```python
from build123d import *

# Parameters (mm, degrees)
SKETCH1_W               = 15
SKETCH1_H               = 22
SKETCH1_R               = 1.3
SKETCH1_R_2             = 0.5
BOSS_EXTRUDE1_DEPTH     = 1.55
SKETCH2_W               = 4.3
SKETCH2_H               = 5.2
BOSS_EXTRUDE2_DEPTH     = 1
SKETCH4_W               = 22
SKETCH4_H               = 1.55
BOSS_EXTRUDE3_DEPTH     = 13
SKETCH6_W               = 5
SKETCH6_H               = 20
BOSS_EXTRUDE4_DEPTH     = 2.4
BOSS_EXTRUDE5_START     = -5
SKETCH7_R               = 0.45
BOSS_EXTRUDE5_DEPTH     = 11
LPATTERN1_COUNT         = 4
LPATTERN1_PITCH         = 2.54
LPATTERN1_COUNT_DIR2    = 2
LPATTERN1_PITCH_DIR2    = 2.54
MIRROR1_START           = -5
MIRROR1_COPY_1_SKETCH_R = 0.45
MIRROR1_COPY_1_DEPTH    = 11
MIRROR1_COPY_2_SKETCH_R = 0.45
MIRROR1_COPY_2_DEPTH    = 11
MIRROR1_COPY_3_SKETCH_R = 0.45
MIRROR1_COPY_3_DEPTH    = 11
MIRROR1_COPY_4_SKETCH_R = 0.45
MIRROR1_COPY_4_DEPTH    = 11
MIRROR1_COPY_5_SKETCH_R = 0.45
MIRROR1_COPY_5_DEPTH    = 11
MIRROR1_COPY_6_SKETCH_R = 0.45
MIRROR1_COPY_6_DEPTH    = 11
MIRROR1_COPY_7_SKETCH_R = 0.45
MIRROR1_COPY_7_DEPTH    = 11


with BuildPart() as part:
    # Sketch1 → Boss-Extrude1 (new body)
    with BuildSketch(Plane(origin=(0, 0, 0), x_dir=(1, 0, 0), z_dir=(0, 1, 0))):
        Rectangle(SKETCH1_W, SKETCH1_H)
        with Locations(Location((-5.5, 9, 0), (0, 0, 90))):
            Circle(SKETCH1_R, mode=Mode.SUBTRACT)
        with Locations(Location((5.5, 9, 0), (0, 0, 90))):
            Circle(SKETCH1_R, mode=Mode.SUBTRACT)
        with Locations(Location((5.5, -9, 0), (0, 0, 90))):
            Circle(SKETCH1_R, mode=Mode.SUBTRACT)
        with Locations(Location((-5.5, -9, 0), (0, 0, 90))):
            Circle(SKETCH1_R, mode=Mode.SUBTRACT)
        with Locations(Location((0, 0, 0), (0, 0, 270))):
            Circle(SKETCH1_R_2, mode=Mode.SUBTRACT)
    extrude(amount=BOSS_EXTRUDE1_DEPTH)

    # Sketch2 → Boss-Extrude2 (add)
    with BuildSketch(Plane(origin=(0, 1.55, 0), x_dir=(1, 0, 0), z_dir=(0, 1, 0))):
        Rectangle(SKETCH2_W, SKETCH2_H)
    extrude(amount=BOSS_EXTRUDE2_DEPTH)

    # Sketch4 → Boss-Extrude3 (add)
    with BuildSketch(Plane(origin=(7.5, 0, 0), x_dir=(0, 0, -1), z_dir=(1, 0, 0))):
        with Locations((0, 0.775)):
            Rectangle(SKETCH4_W, SKETCH4_H)
    extrude(amount=BOSS_EXTRUDE3_DEPTH)

    # Sketch6 → Boss-Extrude4 (add)
    with BuildSketch(Plane.XZ):
        with Locations((16.5, 0)):
            Rectangle(SKETCH6_W, SKETCH6_H)
    extrude(amount=BOSS_EXTRUDE4_DEPTH)

    # Sketch7 → Boss-Extrude5 (add)
    with BuildSketch(Plane.XZ.offset(2.4).offset(BOSS_EXTRUDE5_START)):
        with Locations(Location((15.23, 1.27, 0), (0, 0, 270))):
            Circle(SKETCH7_R)
    boss_extrude5 = extrude(amount=BOSS_EXTRUDE5_DEPTH)

    # LPattern1: Boss-Extrude5 4 × 2
    with Locations(*[(j * LPATTERN1_PITCH_DIR2, 0, i * LPATTERN1_PITCH) for i in range(LPATTERN1_COUNT) for j in range(LPATTERN1_COUNT_DIR2) if (i, j) != (0, 0)]):
        add(boss_extrude5)

    # Mirror1: Boss-Extrude5 across plane
    add(boss_extrude5.mirror(Plane.XY))

    # Mirror1 copy 1 sketch → Mirror1 copy 1 (add)
    with BuildSketch(Plane(origin=(2.54, -2.4, 0), x_dir=(1, 0, 0), z_dir=(0, -1, 0)).offset(MIRROR1_START)):
        with Locations((15.23, -1.27)):
            Circle(MIRROR1_COPY_1_SKETCH_R)
    extrude(amount=MIRROR1_COPY_1_DEPTH)

    # Mirror1 copy 2 sketch → Mirror1 copy 2 (add)
    with BuildSketch(Plane(origin=(0, -2.4, -2.54), x_dir=(1, 0, 0), z_dir=(0, -1, 0)).offset(MIRROR1_START)):
        with Locations((15.23, -1.27)):
            Circle(MIRROR1_COPY_2_SKETCH_R)
    extrude(amount=MIRROR1_COPY_2_DEPTH)

    # Mirror1 copy 3 sketch → Mirror1 copy 3 (add)
    with BuildSketch(Plane(origin=(2.54, -2.4, -2.54), x_dir=(1, 0, 0), z_dir=(0, -1, 0)).offset(MIRROR1_START)):
        with Locations((15.23, -1.27)):
            Circle(MIRROR1_COPY_3_SKETCH_R)
    extrude(amount=MIRROR1_COPY_3_DEPTH)

    # Mirror1 copy 4 sketch → Mirror1 copy 4 (add)
    with BuildSketch(Plane(origin=(0, -2.4, -5.08), x_dir=(1, 0, 0), z_dir=(0, -1, 0)).offset(MIRROR1_START)):
        with Locations((15.23, -1.27)):
            Circle(MIRROR1_COPY_4_SKETCH_R)
    extrude(amount=MIRROR1_COPY_4_DEPTH)

    # Mirror1 copy 5 sketch → Mirror1 copy 5 (add)
    with BuildSketch(Plane(origin=(2.54, -2.4, -5.08), x_dir=(1, 0, 0), z_dir=(0, -1, 0)).offset(MIRROR1_START)):
        with Locations((15.23, -1.27)):
            Circle(MIRROR1_COPY_5_SKETCH_R)
    extrude(amount=MIRROR1_COPY_5_DEPTH)

    # Mirror1 copy 6 sketch → Mirror1 copy 6 (add)
    with BuildSketch(Plane(origin=(0, -2.4, -7.62), x_dir=(1, 0, 0), z_dir=(0, -1, 0)).offset(MIRROR1_START)):
        with Locations((15.23, -1.27)):
            Circle(MIRROR1_COPY_6_SKETCH_R)
    extrude(amount=MIRROR1_COPY_6_DEPTH)

    # Mirror1 copy 7 sketch → Mirror1 copy 7 (add)
    with BuildSketch(Plane(origin=(2.54, -2.4, -7.62), x_dir=(1, 0, 0), z_dir=(0, -1, 0)).offset(MIRROR1_START)):
        with Locations((15.23, -1.27)):
            Circle(MIRROR1_COPY_7_SKETCH_R)
    extrude(amount=MIRROR1_COPY_7_DEPTH)


solid = part.part
```
Part model, mm, in its own coordinate system. A direction names the side the tool comes from. Give positions to 0.01 mm unless a question says otherwise; leave off trailing zeros. Loops run counter-clockwise (first coordinate to the right, second up) from the corner with the lowest first, then second, coordinate; pieces in that order, holes last. Notation, with made-up numbers: M 22,61 L 80,61 A15 ccw 80,76 Z; hole C -19.5,-22 d6. An arc over 180 degrees is marked long. Return JSON: item names as keys, results as strings.
1) 3-axis set-ups, long thin cutter, end or side, ignore diameter. For faces 4 (the face through (15.659, -5.358, -3.675)), 5 (the face through (15.676, 2.082, 8.949)), 6 (the face through (-2.15, 2, 0)): which of +Z, -Z, +X, -X, +Y, -Y reach the whole face in a straight line?
Calculated:
{"face 4": "-Y", "face 5": "+Y", "face 6": "+Z, -Z, -X, +Y"}
2) Saw through at A-A, the plane y = 2.25. Count the separate pieces of the cut face and the enclosed holes in it, then the cut area to 3 significant figures.
Calculated:
{"separate pieces": "17", "enclosed holes": "0", "area": "32.5 mm2"}
3) Pull direction X, two halves, no side cores. Call faces 1 (the face through (15.676, 2.082, 1.329)), 2 (the face through (19, -1, 0)), 3 (the face through (17.8, -8.4, -6.3)): released by +X, released by -X, zero draft, split by the parting line, or undercut.
Calculated:
{"face 1": "undercut", "face 2": "released by +X", "face 3": "zero draft"}
4) Flat gauge pins, fed straight in: pin 1 Ø0.8 at (x, z) = (0, 0) entering from -Y; pin 2 Ø2 at (x, z) = (-4.5, 8.5) entering from +Y; pin 3 Ø4.5 at (x, z) = (0.5, -0.5) entering from +Y. Where does each tip first touch, or does it go through?
Calculated:
{"pin 1": "stops at y = 1.55", "pin 2": "stops at y = 1.55", "pin 3": "stops at y = 2.55"}
5) Saw through at D-D, the plane z = 0. List the corners of the cut face in (x, y).
Calculated:
{"outline": "M -7.5,0 L -0.5,0 L -0.5,1.55 L 0.5,1.55 L 0.5,0 L 14,0 L 14,-2.4 L 19,-2.4 L 19,0 L 20.5,0 L 20.5,1.55 L 2.15,1.55 L 2.15,2.55 L -2.15,2.55 L -2.15,1.55 L -7.5,1.55 Z"}
6) Drill centre lines: line 1 (Z direction, x = -5.5, y = 1.15); line 2 (X direction, y = 0.75, z = -9); line 3 (X direction, y = 0.85, z = 0). Where is each one in solid material? Low to high.
Calculated:
{"line 1": "z = -11 to -10.3, -7.7 to 7.7, 10.3 to 11", "line 2": "x = -7.5 to -6.8, -4.2 to 4.2, 6.8 to 20.5", "line 3": "x = -7.5 to -0.5, 0.5 to 20.5"}
